Autodesk Inventor part; units mm, degrees
ref_plane "dia1_XY" through (0, 2.3749, 0) normal (1, 0, 0) x (0, 0, -1)
ref_plane "dia1_YZ" through (0, 2.3749, 0) normal (0, 0, -1) x (0, 1, 0)
ref_plane "dia1_ZX" through (0, 2.3749, 0) normal (0, 1, 0) x (1, 0, 0)
sketch "Sketch_1" plane through (0, 0, 0) normal (0, 0, 1) x (1, 0, 0)
  line L0 (70.5866, 0) -> (0, 0)
  line L1 (0, 0) -> (0, 2.3749)
  line L2 (0, 2.3749) -> (54.7624, 2.3749)
  line L3 (54.7624, 2.3749) -> (54.7624, 7.22)
  line L4 (54.7624, 7.22) -> (70.5866, 7.22)
  line L5 (70.5866, 7.22) -> (70.5866, 0)
  line L6 (70.5866, 0) -> (0, 0)
revolve "Revolution1" add sketch "Sketch_1" angle 360 about axis through (70.5866, 0, 0) along (1, 0, 0)
sketch "Sketch_3" plane through (0, 0, 0) normal (0, 0, 1) x (1, 0, 0)
  line L0 (0, 0) -> (-12.7, 0)
  line L1 (-12.7, 0) -> (-12.7, 1.9406)
  line L2 (-12.7, 1.9406) -> (-12.2276, 2.413)
  line L3 (-12.2276, 2.413) -> (0, 2.413)
  line L4 (0, 2.413) -> (0, 0)
  line L5 (0, 0) -> (-12.7, 0)
revolve "Revolution2" add sketch "Sketch_3" angle 360 about axis through (0, 0, 0) along (1, 0, 0)
thread "Thread1"
sketch "Sketch_30" plane through (0, 0, 0) normal (0, 0, 1) x (1, 0, 0)
  line L0 (0, 0) -> (-0.254, 0)
  line L1 (-0.254, 2.159) -> (0, 2.159)
  line L2 (0, 2.159) -> (0, 2.667)
  line L3 (0, 2.667) -> (-0.254, 2.667)
  line L4 (-0.254, 2.667) -> (-0.254, 2.159)
revolve "Revolution3" cut sketch "Sketch_30" angle 360 about axis through (0, 0, 0) along (1, 0, 0)
ref_plane "dia1_XY" through (0, 2.3749, 0) normal (1, 0, 0) x (0, 0, -1)
ref_plane "dia1_YZ" through (0, 2.3749, 0) normal (0, 0, -1) x (0, 1, 0)
ref_plane "dia1_ZX" through (0, 2.3749, 0) normal (0, 1, 0) x (1, 0, 0)
ref_plane "dia12_XY" through (0, 0, 7.8105) normal (1, 0, 0) x (0, 0, -1)
ref_plane "dia12_YZ" through (0, 0, 7.8105) normal (0, 0, -1) x (0, 1, 0)
ref_plane "dia12_ZX" through (0, 0, 7.8105) normal (0, 1, 0) x (1, 0, 0)
ref_plane "dia2_XY" through (0, -2.3749, 0) normal (1, 0, 0) x (0, 0, -1)
ref_plane "dia2_YZ" through (0, -2.3749, 0) normal (0, 0, -1) x (0, 1, 0)
ref_plane "dia2_ZX" through (0, -2.3749, 0) normal (0, 1, 0) x (1, 0, 0)
ref_plane "dia22_XY" through (0, 0, -7.8105) normal (1, 0, 0) x (0, 0, -1)
ref_plane "dia22_YZ" through (0, 0, -7.8105) normal (0, 0, -1) x (0, 1, 0)
ref_plane "dia22_ZX" through (0, 0, -7.8105) normal (0, 1, 0) x (1, 0, 0)
ref_plane "rl1_XY" through (-12.7, 0, 0) normal (1, 0, 0) x (0, 0, -1)
ref_plane "rl1_YZ" through (-12.7, 0, 0) normal (0, 0, -1) x (0, 1, 0)
ref_plane "rl1_ZX" through (-12.7, 0, 0) normal (0, 1, 0) x (1, 0, 0)
ref_plane "rl2_XY" through (0, 0, 0) normal (1, 0, 0) x (0, 0, -1)
ref_plane "rl2_YZ" through (0, 0, 0) normal (0, 0, -1) x (0, 1, 0)
ref_plane "rl2_ZX" through (0, 0, 0) normal (0, 1, 0) x (1, 0, 0)
ref_plane "rod_cp_XY" through (0, 0, 0) normal (1, 0, 0) x (0, 0, -1)
ref_plane "rod_cp_YZ" through (0, 0, 0) normal (0, 0, -1) x (0, 1, 0)
ref_plane "rod_cp_ZX" through (0, 0, 0) normal (0, 1, 0) x (1, 0, 0)
ref_plane "thd1_XY" through (-12.7, 2.413, 0) normal (1, 0, 0) x (0, 0, -1)
ref_plane "thd1_YZ" through (-12.7, 2.413, 0) normal (0, 0, -1) x (0, 1, 0)
ref_plane "thd1_ZX" through (-12.7, 2.413, 0) normal (0, 1, 0) x (1, 0, 0)
ref_plane "thd2_XY" through (-12.7, -2.413, 0) normal (1, 0, 0) x (0, 0, -1)
ref_plane "thd2_YZ" through (-12.7, -2.413, 0) normal (0, 0, -1) x (0, 1, 0)
ref_plane "thd2_ZX" through (-12.7, -2.413, 0) normal (0, 1, 0) x (1, 0, 0)
ref_plane "to_rod_clevis_XY" through (-12.7, 0, 0) normal (1, 0, 0) x (0, 0, -1)
ref_plane "to_rod_clevis_YZ" through (-12.7, 0, 0) normal (0, 0, -1) x (0, 1, 0)
ref_plane "to_rod_clevis_ZX" through (-12.7, 0, 0) normal (0, 1, 0) x (1, 0, 0)
properties part number "021-DXP0000_rod"
Here's how the part is built. I have some questions about the finished solid (model axes, mm). Coordinates: 2 decimals unless noted, no trailing zeros. Loops run counter-clockwise (first coordinate to the right, second up) from the corner with the lowest first, then second, coordinate; pieces in that order, holes last. Notation, with made-up numbers: M 54.5,-4 L 93.5,-4 A19 cw 93.5,10 Z; hole C -11,74 d1. An arc over 180 degrees is marked long. One line per item, written item: value.
1. Imagine slicing it at C-C (x = 21). List the corners of the cut face in (y, z) for me, and give its area (3 significant figures).
Geometry says:
outline: C 0,0 d4.75
area: 17.7 mm2
2. Imagine slicing it at A-A (y = 0). List the corners of the cut face in (x, z) for me.
Geometry says:
outline: M -12.7,-1.94 L -12.23,-2.41 L -0.25,-2.41 L -0.25,-2.16 L 0,-2.16 L 0,-2.37 L 54.76,-2.37 L 54.76,-7.22 L 70.59,-7.22 L 70.59,7.22 L 54.76,7.22 L 54.76,2.37 L 0,2.37 L 0,2.16 L -0.25,2.16 L -0.25,2.41 L -12.23,2.41 L -12.7,1.94 Z
3. Will these pins go through, and if not, where does the flat tip stop? pin 1 Ø6 at (x, z) = (52.5, -3) entering from -Y; pin 2 Ø1.5 at (y, z) = (-3, 1.5) entering from -X; pin 3 Ø3 at (x, y) = (59, 5) entering from -Z.
Geometry says:
pin 1: stops at y = -7.15
pin 2: stops at x = 54.76
pin 3: stops at z = -6.31
4. Please list where these lines run through material, in increasing order: probe 1 along X at (y, z) = (-3.5, 0.75); probe 2 along Z at (x, y) = (5.5, 0); probe 3 along Y at (x, z) = (-6, -0.25).
Geometry says:
probe 1: x = 54.76 to 70.59
probe 2: z = -2.37 to 2.37
probe 3: y = -2.4 to 2.4
5. Imagine slicing it at D-D (x = 60). List the corners of the cut face in (y, z) for me, and give its area (3 significant figures).
Geometry says:
outline: C 0,0 d14.44
area: 164 mm2
